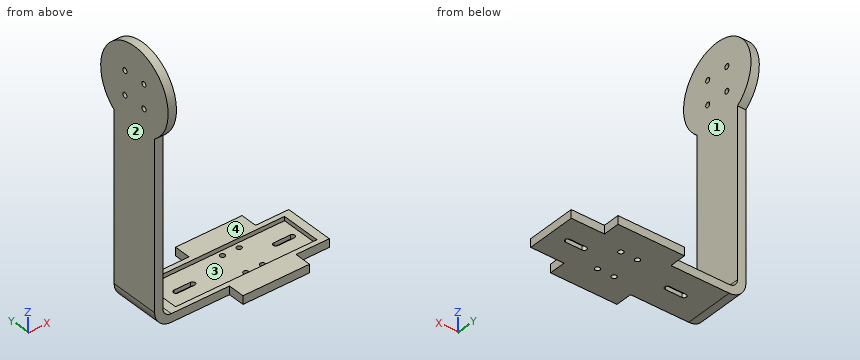
```python
from build123d import *

# Parameters (mm, degrees)
BOSS_EXTRUDE1_DEPTH = 30
SKETCH4_R           = 25
BOSS_EXTRUDE3_DEPTH = 5
SKETCH8_W           = 85
SKETCH8_H           = 24
CUT_EXTRUDE2_DEPTH  = 2.5
SKETCH11_R          = 1.5
CUT_EXTRUDE4_DEPTH  = 5
SKETCH12_W          = 40
SKETCH12_H          = 10
BOSS_EXTRUDE5_DEPTH = 5
CUT_EXTRUDE5_DEPTH  = 2.5
SKETCH14_R          = 1.5
CUT_EXTRUDE6_DEPTH  = 189.745860882


with BuildPart() as part:
    # Sketch1 → Boss-Extrude1 (new body)
    with BuildSketch(Plane(origin=(0, 0, 0), x_dir=(1, 0, 0), z_dir=(0, 1, 0))):
        with BuildLine():
            Line((0, -5), (0, -125))
            Line((0, -125), (-5, -125))
            Line((-5, -125), (-5, -5))
            ThreePointArc((-5, -5), (-2.071067812, 2.071067812), (5, 5))
            Line((5, 5), (100, 5))
            Line((100, 5), (100, 0))
            Line((100, 0), (5, 0))
            ThreePointArc((5, 0), (1.464466094, -1.464466094), (0, -5))
        make_face()
    extrude(amount=-BOSS_EXTRUDE1_DEPTH)

    # Sketch4 → Boss-Extrude3 (add)
    with BuildSketch(Plane(origin=(0, 0, 0), x_dir=(0, 0, -1), z_dir=(1, 0, 0))):
        with Locations((-125, -15)):
            Circle(SKETCH4_R)
    extrude(amount=-BOSS_EXTRUDE3_DEPTH)

    # Sketch8 → Cut-Extrude2 (cut)
    with BuildSketch(Plane.XY):
        with Locations((52.5, -15)):
            Rectangle(SKETCH8_W, SKETCH8_H)
    extrude(amount=-CUT_EXTRUDE2_DEPTH, mode=Mode.SUBTRACT)

    # Sketch11 → Cut-Extrude4 (cut)
    with BuildSketch(Plane.ZY.offset(5)):
        with Locations((132.071067812, -7.928932188)):
            Circle(SKETCH11_R)
        with Locations((132.071067812, -22.071067812)):
            Circle(SKETCH11_R)
        with Locations((117.928932188, -22.071067812)):
            Circle(SKETCH11_R)
        with Locations((117.928932188, -7.928932188)):
            Circle(SKETCH11_R)
    extrude(amount=-CUT_EXTRUDE4_DEPTH, mode=Mode.SUBTRACT)

    # Sketch12 → Boss-Extrude5 (add)
    with BuildSketch(Plane(origin=(0, 0, -5), x_dir=(-1, 0, 0), z_dir=(0, 0, -1))):
        with Locations((-60, 5)):
            Rectangle(SKETCH12_W, SKETCH12_H)
        with Locations((-60, -35)):
            Rectangle(SKETCH12_W, SKETCH12_H)
    extrude(amount=-BOSS_EXTRUDE5_DEPTH)

    # Sketch13 → Cut-Extrude5 (cut)
    with BuildSketch(Plane.XY.offset(-2.5)):
        with BuildLine():
            Line((90, -16.5), (80, -16.5))
            ThreePointArc((80, -16.5), (78.5, -15), (80, -13.5))
            Line((80, -13.5), (90, -13.5))
            ThreePointArc((90, -13.5), (91.5, -15), (90, -16.5))
        make_face()
        with BuildLine():
            Line((20, -16.5), (30, -16.5))
            ThreePointArc((30, -16.5), (31.5, -15), (30, -13.5))
            Line((30, -13.5), (20, -13.5))
            ThreePointArc((20, -13.5), (18.5, -15), (20, -16.5))
        make_face()
    extrude(amount=-CUT_EXTRUDE5_DEPTH, mode=Mode.SUBTRACT)

    # Sketch14 → Cut-Extrude6 (cut, through all)
    with BuildSketch(Plane(origin=(0, 0, -5), x_dir=(-1, 0, 0), z_dir=(0, 0, -1))):
        with Locations((-65, -6.339745962)):
            Circle(SKETCH14_R)
        with Locations((-55, -6.339745962)):
            Circle(SKETCH14_R)
        with Locations((-55, -23.660254038)):
            Circle(SKETCH14_R)
        with Locations((-65, -23.660254038)):
            Circle(SKETCH14_R)
    extrude(amount=-CUT_EXTRUDE6_DEPTH, mode=Mode.SUBTRACT)


solid = part.part
```
Geometry check sheet. Reference: the model listing, model coordinates, mm. Face numbers are marked on the shaded views. A direction names the side the tool comes from. Coordinates: 2 decimals unless noted, no trailing zeros. Write each loop counter-clockwise with the first axis right and the second up, starting at its lowest first coordinate (ties: lowest second). Pieces come first, ordered by that corner, then holes. Notation, with made-up numbers: (58, 55) -> (93, 55) arc R27 cw to (93, 83) -> close; hole circle Ø4 at (32, 72.5). An arc over 180 degrees is marked (long way). Use CSV: the item, a comma, the result in double quotes. Start each with the question number.
Item 1: Set-up check for the marked faces 1 and 2: record each of +Z, -Z, +X, -X, +Y, -Y from which the full face is reachable in a straight line by a thin tool's end or side.
Item 2: Cross-section at B-B, the plane x = 61.5. Record the cut outline in (y, z).
Item 3: Thickness scan on line 1 (Y direction, x = 65, z = -4.1); line 2 (Z direction, x = 15, y = -24.5); line 3 (Z direction, x = 54.5, y = -28). Record the ranges inside material, lowest first.
Item 4: Cross-section at C-C, the plane y = 7. Record the cut outline in (x, z).
Item 5: Depth check by flat-ended pin: pin 1 Ø1.5 at (y, z) = (-33.5, -3) entering from -X; pin 2 Ø10 at (y, z) = (-26, 81.5) entering from +X; pin 3 Ø2.5 at (x, z) = (94, -3.5) entering from +Y. Enter the tip coordinate at first touch or a pass-through.
Item 6: Cross-section at A-A, the plane x = 86. Record the cut outline in (y, z).
Item 7: Mould release check, pull along Y, two halves, no side actions. Record for the marked faces 3 and 4: released by +Y, released by -Y, zero draft, split by the parting line, or undercut.
Item 8: Cross-section at D-D, the plane z = 21. Record the cut outline in (x, y), plus the area to 3 significant figures.
Answers:
1,face 1,"+Z, +X, +Y, -Y"
1,face 2,"+Z, -Z, -X, +Y, -Y"
2,outline,"(-40, -5) -> (10, -5) -> (10, 0) -> (-3, 0) -> (-3, -2.5) -> (-27, -2.5) -> (-27, 0) -> (-40, 0) -> close"
3,line 1,"-40 to -25.16, -22.16 to -7.84, -4.84 to 10"
3,line 2,"-5 to -2.5"
3,line 3,"-5 to 0"
4,outline,"(-5, 113.13) -> (0, 113.13) -> (0, 136.87) -> (-5, 136.87) -> close; (40, -5) -> (80, -5) -> (80, 0) -> (40, 0) -> close"
5,pin 1,"x = 40"
5,pin 2,"x = 0"
5,pin 3,"y = 0"
6,outline,"(-30, -5) -> (-16.5, -5) -> (-16.5, -2.5) -> (-27, -2.5) -> (-27, 0) -> (-30, 0) -> close; (-13.5, -5) -> (0, -5) -> (0, 0) -> (-3, 0) -> (-3, -2.5) -> (-13.5, -2.5) -> close"
7,face 3,"undercut"
7,face 4,"zero draft"
8,outline,"(-5, -30) -> (0, -30) -> (0, 0) -> (-5, 0) -> close"
8,area,"150 mm^2"
